Part model, mm, in its own coordinate system. A direction names the side the tool comes from. Round coordinates to 2 decimals unless told otherwise and drop trailing zeros. Order: outer loops, then holes, each group sorted by start corner. A loop starts at its lowest first (then second) coordinate and runs counter-clockwise, first axis right, second up. Notation, with made-up numbers: (53.5, 38) - (108.5, 38) arc R19 ccw to (108.5, 65) - close; hole circle Ø9 at (49.25, 47). An arc over 180 degrees is marked (long way). Answer as a JSON object with one key per item and string values.
```python
from build123d import *

# Parameters (mm, degrees)
ESTRUSIONE_ESTRUSIONE1_DEPTH = 9
FORO_8_0_8_1_D               = 8


with BuildPart() as part:
    # Schizzo1 → Estrusione-Estrusione1 (new, symmetric)
    with BuildSketch(Plane(origin=(0, 0, 0), x_dir=(1, 0, 0), z_dir=(0, 1, 0))):
        Polygon((30, 16), (-30, 16), (-30, -4), (-20, -14), (-18, -14), (-4, 0), (4, 0), (18, -14), (20, -14), (30, -4), align=None)
    extrude(amount=ESTRUSIONE_ESTRUSIONE1_DEPTH, both=True)

    # Foro Ø8.0 (8)-1 (through all)
    with Locations(Plane(origin=(0, 9, 0), x_dir=(1, 0, 0), z_dir=(0, 1, 0))):
        with Locations((19, 8), (-19, 8)):
            Hole(FORO_8_0_8_1_D / 2)


solid = part.part
```
Item 1: Drop flat-ended pins along their axis: P1, Ø5, axis at x = 8, z = 10.5, coming from the -Y side; P2, Ø1.5, axis at x = -15, y = -1, coming from the +Z side; P3, Ø3, axis at y = 7, z = 6, coming from the -X side; P4, Ø4, axis at x = 1, y = 4.5, coming from the +Z side. Give the stop position or say it passes through.
Taken from the geometry:
{"P1": "through", "P2": "z = 11.75", "P3": "x = -29.5", "P4": "z = 0"}
Item 2: Cut at A-A (z = -8). Write the cut outline in (x, y), plus the area to 3 significant figures.
Taken from the geometry:
{"outline": "(-30, -9) - (-23, -9) - (-23, 9) - (-30, 9) - close; (-15, -9) - (15, -9) - (15, 9) - (-15, 9) - close; (23, -9) - (30, -9) - (30, 9) - (23, 9) - close", "area": "792 mm2"}
Item 3: Probe L1, parallel to Z at x = 19, y = 2.25; L2, parallel to X at y = -4, z = -8.5; L3, parallel to X at y = 5.75, z = 10. List the from-to ranges inside material, lowest first. Write a range as from..to.
Taken from the geometry:
{"L1": "-16..-12, -4..14", "L2": "-30..-22.97, -15.03..15.03, 22.97..30", "L3": "-24..-14, 14..24"}
Item 4: Tool access for faces 5 (the flat face through (30, 0, -6)), 6 (the flat face through (0, 0, 0)): list every direction of +Z, -Z, +X, -X, +Y, -Y with a clear straight run to the whole face (end or side of a thin tool).
Taken from the geometry:
{"face 5": "+Z, -Z, +X, +Y, -Y", "face 6": "+Z, +Y, -Y"}
Item 5: Two-plate mould, pull along Z, no slides. Class faces 1 (the flat face through (0, 0, -16)), 2 (the flat face through (0, 9, -5)), 3 (the cylindrical face through (-18.133, -0.126, -4.095)), 4 (the cylindrical face through (19.867, -0.126, -4.095)): pulls with the +Z half, pulls with the -Z half, needs draft (parallel to the pull), parting line crosses it, or undercut.
Taken from the geometry:
{"face 1": "pulls with the -Z half", "face 2": "needs draft", "face 3": "undercut", "face 4": "undercut"}
Item 6: Cut at D-D (z = 2.5). Write the cut outline in (x, y), plus the area to 3 significant figures.
Taken from the geometry:
{"outline": "(-30, -9) - (-6.5, -9) - (-6.5, 9) - (-30, 9) - close; (6.5, -9) - (30, -9) - (30, 9) - (6.5, 9) - close", "area": "846 mm2"}
Item 7: Cut at C-C (x = 21.5). Write the cut outline in (y, z).
Taken from the geometry:
{"outline": "(-9, -16) - (9, -16) - (9, -11.12) - (-9, -11.12) - close; (-9, -4.88) - (9, -4.88) - (9, 12.5) - (-9, 12.5) - close"}
Item 8: Cut at B-B (y = -6.5). Write the cut outline in (x, z), plus the area to 3 significant figures.
Taken from the geometry:
{"outline": "(-30, -16) - (30, -16) - (30, 4) - (20, 14) - (18, 14) - (4, 0) - (-4, 0) - (-18, 14) - (-20, 14) - (-30, 4) - close; hole circle Ø8 at (-19, -8); hole circle Ø8 at (19, -8)", "area": "1,290 mm2"}
